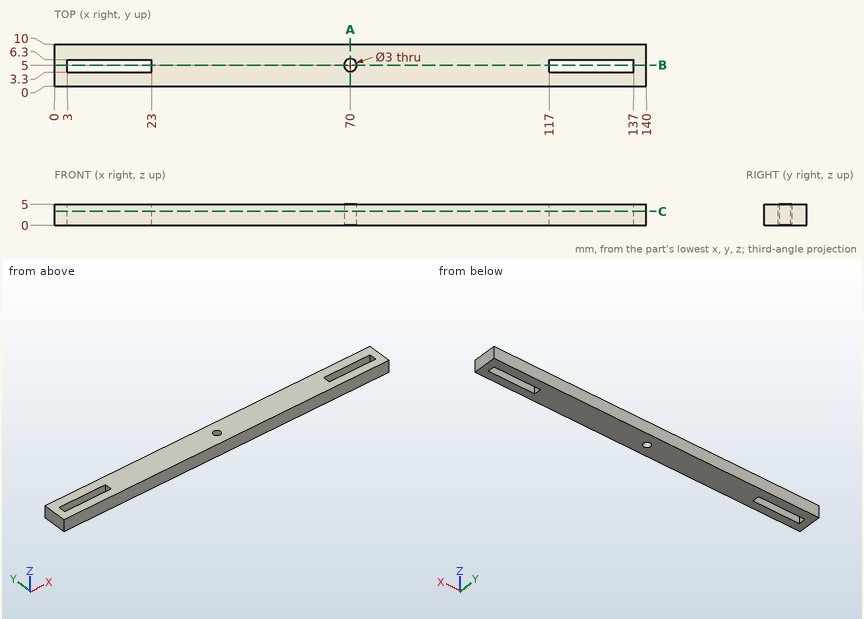
Print and shaded views of the part. All mm, measured from the part's lowest x, y and z. Round coordinates to 2 decimals unless told otherwise and drop trailing zeros. Order: outer loops, then holes, each group sorted by start corner. A loop starts at its lowest first (then second) coordinate and runs counter-clockwise, first axis right, second up. Notation, with made-up numbers: (53.25, 59.25) - (57.25, 59.25) arc R19 ccw to (57.25, 96.25) - close; hole circle Ø7 at (26, 35.25). An arc over 180 degrees is marked (long way). Use a Markdown table: item, result.
1) Saw through at C-C on z = 3.3. Write the cut outline in (x, y).
Recorded:
| item | result |
|---|---|
| outline | (0, 0) - (140, 0) - (140, 10) - (0, 10) - close; hole (3, 3.3) - (23, 3.3) - (23, 6.3) - (3, 6.3) - close; hole circle Ø3 at (70, 5); hole (117, 3.3) - (137, 3.3) - (137, 6.3) - (117, 6.3) - close |
2) Saw through at A-A on x = 70. Write the cut outline in (y, z), and give its area (3 significant figures).
Recorded:
| item | result |
|---|---|
| outline | (0, 0) - (3.5, 0) - (3.5, 5) - (0, 5) - close; (6.5, 0) - (10, 0) - (10, 5) - (6.5, 5) - close |
| area | 35.0 mm² |
3) Saw through at B-B on y = 5. Write the cut outline in (x, z), and give its area (3 significant figures).
Recorded:
| item | result |
|---|---|
| outline | (0, 0) - (3, 0) - (3, 5) - (0, 5) - close; (23, 0) - (68.5, 0) - (68.5, 5) - (23, 5) - close; (71.5, 0) - (117, 0) - (117, 5) - (71.5, 5) - close; (137, 0) - (140, 0) - (140, 5) - (137, 5) - close |
| area | 485 mm² |
4) Wall check: L1, parallel to X at y = 5.25, z = 2.05; L2, parallel to Y at x = 70, z = 2; L3, parallel to Y at x = 19, z = 4.4. Give the ranges that are in metal, low to high.
Recorded:
| item | result |
|---|---|
| L1 | x = 0 to 3, 23 to 68.52, 71.48 to 117, 137 to 140 |
| L2 | y = 0 to 3.5, 6.5 to 10 |
| L3 | y = 0 to 3.3, 6.3 to 10 |
